Answer from the drawing. Dimensions are ordinates in mm from the lowest x, y and z of the part. A direction names the side the tool comes from. Coordinates: 2 decimals unless noted, no trailing zeros. Write each loop counter-clockwise with the first axis right and the second up, starting at its lowest first coordinate (ties: lowest second). Pieces come first, ordered by that corner, then holes. Notation, with made-up numbers: (20.25, 28) - (57.25, 28) arc R18 cw to (57.25, 40) - close; hole circle Ø8 at (-17.5, -15). An arc over 180 degrees is marked (long way). Use CSV: the item, a comma, the result in double quotes. Start each with the question number.
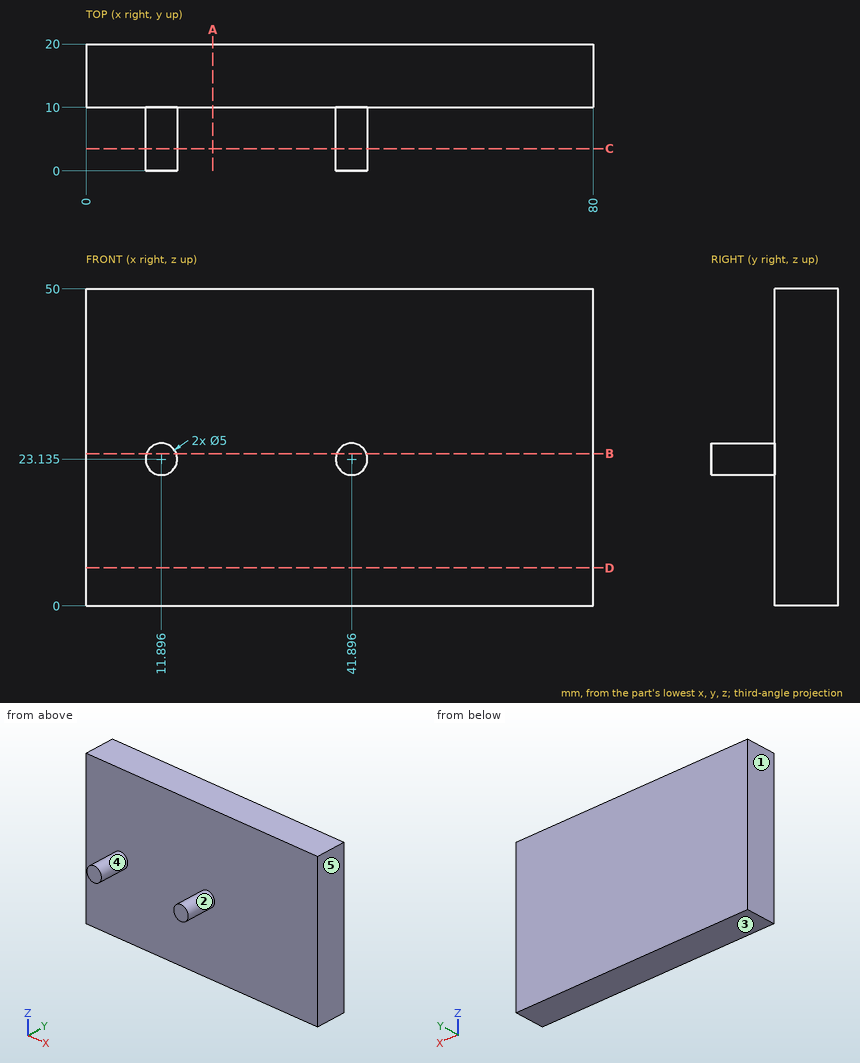
Item 1: A cutting plane is placed at A-A (x = 20). Determine the outline of the cut face in (y, z), then the cut area to 3 significant figures.
Item 2: A cutting plane is placed at C-C (y = 3.5). Determine the outline of the cut face in (x, z) (1 decimal).
Item 3: Straight lines are drawn through the part: probe 1 along Y at (x, z) = (59, 22); probe 2 along X at (y, z) = (3.5, 24). For each, find the intervals that lie inside material, in ascending order. Write a range as [from, to].
Item 4: Each of these flat-tipped pins is pushed along its axis until it touches: pin 1 (2 mm diameter, centred on y = 5, z = 20.5, fed in from +X); pin 2 (12 mm diameter, centred on y = 3.5, z = 13.5, fed in from -X); pin 3 (8 mm diameter, centred on y = 5.5, z = 26.5, fed in from +X); pin 4 (12 mm diameter, centred on x = 35, z = 39.5, fed in from -Y). Where does it stop, or does it pass through?
Item 5: A cutting plane is placed at B-B (z = 24). Determine the outline of the cut face in (x, y), then the cut area to 3 significant figures.
Item 6: Which of the six approach directions +Z, -Z, +X, -X, +Y, -Y give full straight-line access (tool end or side, diameter ignored) to the marked faces 4 and 5?
Item 7: Determine the mould class of the marked faces 1, 2 and 3 for opening direction X: +X half, -X half, draft (parallel to the pull), parting line (faces both ways), or undercut.
Item 8: A cutting plane is placed at D-D (z = 6). Determine the outline of the cut face in (x, y), then the cut area to 3 significant figures.
Calculated:
1,outline,"(10, 0) - (20, 0) - (20, 50) - (10, 50) - close"
1,area,"500 mm²"
2,outline,"circle Ø5 at (11.9, 23.1); circle Ø5 at (41.9, 23.1)"
3,probe 1,"y = [10, 20]"
3,probe 2,"x = [9.55, 14.24], [39.55, 44.24]"
4,pin 1,"stops at x = 43.79"
4,pin 2,"passes through"
4,pin 3,"stops at x = 44.4"
4,pin 4,"stops at y = 10"
5,outline,"(0, 10) - (9.55, 10) - (9.55, 0) - (14.24, 0) - (14.24, 10) - (39.55, 10) - (39.55, 0) - (44.24, 0) - (44.24, 10) - (80, 10) - (80, 20) - (0, 20) - close"
5,area,"894 mm²"
6,face 4,"-Y"
6,face 5,"+Z, -Z, +X, +Y, -Y"
7,face 1,"-X half"
7,face 2,"undercut"
7,face 3,"draft"
8,outline,"(0, 10) - (80, 10) - (80, 20) - (0, 20) - close"
8,area,"800 mm²"
